Read the model definition and answer for the solid it produces. Units are mm, in the model's axes. A direction names the side the tool comes from. Coordinates: 2 decimals unless noted, no trailing zeros. Write each loop counter-clockwise with the first axis right and the second up, starting at its lowest first coordinate (ties: lowest second). Pieces come first, ordered by that corner, then holes. Notation, with made-up numbers: (-29.5, -37.5) -> (-6.5, -37.5) arc R20 cw to (-6.5, -15.5) -> close; hole circle Ø5 at (65, 37.5). An arc over 180 degrees is marked (long way). Answer as a JSON object with one key per item and string values. Group by question number.
(1) Find section A-A (z = 10.5). Give the vertices of the cut face in (x, y) (3 decimals), then the cut area to 3 significant figures.
(2) For a pull along X with two mould halves and no side action, classify faces 5 (the face through (-282.92, -76.1, 79.81)), 6 (the face through (-329.875, -83, 80)), 7 (the face through (-221.025, -83, 57)), 8 (the face through (-263.066, -87.263, 28.924)) as +X half, -X half, draft (parallel to the pull), parting line (faces both ways), or undercut.
(3) Flat-ended cylindrical pins translate along their axes: P1, Ø2, axis at y = -78, z = 43, coming from the +X side (3 decimals); P2, Ø3, axis at x = -256, y = -83, coming from the -Z side; P3, Ø15, axis at x = -290.57, z = 38.77, coming from the -Y side; P4, Ø3, axis at x = -256.5, y = -84, coming from the +Z side. Find the tip coordinate at first contact, or state that the pin passes through.
(4) Which of the six approach directions +Z, -Z, +X, -X, +Y, -Y give full straight-line access (tool end or side, diameter ignored) to faces 1 (the face through (-284, -82, 28.4)), 2 (the face through (-311, -84, 144.63)), 3 (the face through (-257, -82, 20.2)), 4 (the face through (-233.835, -87, 56))?
(5) Find section C-C (x = -275.57). Give the vertices of the cut face in (y, z).
(6) Find section D-D (z = 146.5). Give the vertices of the cut face in (x, y) (3 decimals), then the cut area to 3 significant figures.
(7) Straight lines are drawn through the part: L1, parallel to X at y = -83.75, z = 151 (3 decimals); L2, parallel to X at y = -79, z = 18 (3 decimals); L3, parallel to Z at x = -272.5, y = -84.75. For each, find the intervals that lie inside material, in ascending order.
(8) Find section B-B (x = -290.57). Give the vertices of the cut face in (y, z), then the cut area to 3 significant figures.
from build123d import *

# Parameters (mm, degrees)
SKETCH1_W           = 95.25
SKETCH1_H           = 12.8
BOSS_EXTRUDE1_DEPTH = 161.88
SKETCH1_3_R         = 3.1
CUT_EXTRUDE1_DEPTH  = 20.2
SKETCH1_4_R         = 2.395
CUT_EXTRUDE2_DEPTH  = 21.5
CUT_EXTRUDE3_REACH  = 14.8
SKETCH2_R           = 9.525
SKETCH2_R_2         = 3.265
SKETCH3_R           = 3.265
SKETCH3_R_2         = 9.525
CUT_EXTRUDE4_DEPTH  = 3.32
CUT_EXTRUDE5_START  = -17.25
SKETCH4_R           = 1.965
CUT_EXTRUDE5_DEPTH  = 17.25
SKETCH6_R           = 9.5
CUT_EXTRUDE6_DEPTH  = 13.8000001


with BuildPart() as part:
    # Sketch1 → Boss-Extrude1 (new body)
    with BuildSketch(Plane.XY):
        with Locations((-282.25, -82.5)):
            Rectangle(SKETCH1_W, SKETCH1_H)
    extrude(amount=BOSS_EXTRUDE1_DEPTH)

    # Sketch1<3> → Cut-Extrude1 (cut)
    with BuildSketch(Plane.XY):
        with Locations((-308, -82.5)):
            Circle(SKETCH1_3_R)
        with Locations((-257.2, -82.5)):
            Circle(SKETCH1_3_R)
    extrude(amount=CUT_EXTRUDE1_DEPTH, mode=Mode.SUBTRACT)

    # Sketch1<4> → Cut-Extrude2 (cut)
    with BuildSketch(Plane.XY):
        with Locations((-320.5, -82.5)):
            Circle(SKETCH1_4_R)
        with Locations((-244.2, -82.5)):
            Circle(SKETCH1_4_R)
    extrude(amount=CUT_EXTRUDE2_DEPTH, mode=Mode.SUBTRACT)

    # Sketch2 → Cut-Extrude3 (cut, up to next)
    with BuildSketch(Plane(origin=(0, -76.1, 0), x_dir=(-1, 0, 0), z_dir=(0, 1, 0)), mode=Mode.PRIVATE) as cut_extrude3_sk1:
        with Locations((275.57, 86.105)):
            Circle(SKETCH2_R)
    cut_extrude3_tool1 = extrude(cut_extrude3_sk1.sketch, amount=-CUT_EXTRUDE3_REACH, mode=Mode.PRIVATE) & part.part
    add(cut_extrude3_tool1.solids().sort_by_distance((-275.57, -76.1, 86.105))[0], mode=Mode.SUBTRACT)
    # Sketch2 → Cut-Extrude3 (cut, up to next)
    with BuildSketch(Plane(origin=(0, -76.1, 0), x_dir=(-1, 0, 0), z_dir=(0, 1, 0)), mode=Mode.PRIVATE) as cut_extrude3_sk2:
        with Locations((275.57, 124.135)):
            Circle(SKETCH2_R)
    cut_extrude3_tool2 = extrude(cut_extrude3_sk2.sketch, amount=-CUT_EXTRUDE3_REACH, mode=Mode.PRIVATE) & part.part
    add(cut_extrude3_tool2.solids().sort_by_distance((-275.57, -76.1, 124.135))[0], mode=Mode.SUBTRACT)
    # Sketch2 → Cut-Extrude3 (cut, up to next)
    with BuildSketch(Plane(origin=(0, -76.1, 0), x_dir=(-1, 0, 0), z_dir=(0, 1, 0)), mode=Mode.PRIVATE) as cut_extrude3_sk3:
        with Locations((253.55, 28.505)):
            Circle(SKETCH2_R_2)
    cut_extrude3_tool3 = extrude(cut_extrude3_sk3.sketch, amount=-CUT_EXTRUDE3_REACH, mode=Mode.PRIVATE) & part.part
    add(cut_extrude3_tool3.solids().sort_by_distance((-253.55, -76.1, 28.505))[0], mode=Mode.SUBTRACT)
    # Sketch2 → Cut-Extrude3 (cut, up to next)
    with BuildSketch(Plane(origin=(0, -76.1, 0), x_dir=(-1, 0, 0), z_dir=(0, 1, 0)), mode=Mode.PRIVATE) as cut_extrude3_sk4:
        with Locations((240.925, 140.49)):
            Circle(SKETCH2_R_2)
    cut_extrude3_tool4 = extrude(cut_extrude3_sk4.sketch, amount=-CUT_EXTRUDE3_REACH, mode=Mode.PRIVATE) & part.part
    add(cut_extrude3_tool4.solids().sort_by_distance((-240.925, -76.1, 140.49))[0], mode=Mode.SUBTRACT)
    # Sketch2 → Cut-Extrude3 (cut, up to next)
    with BuildSketch(Plane(origin=(0, -76.1, 0), x_dir=(-1, 0, 0), z_dir=(0, 1, 0)), mode=Mode.PRIVATE) as cut_extrude3_sk5:
        with BuildLine():
            Line((269.505, 25.4), (269.505, 0))
            Line((269.505, 0), (298.155, 0))
            Line((298.155, 0), (298.155, 25.4))
            ThreePointArc((298.155, 25.4), (297.276320344, 27.521320344), (295.155, 28.4))
            Line((295.155, 28.4), (272.505, 28.4))
            ThreePointArc((272.505, 28.4), (270.383679656, 27.521320344), (269.505, 25.4))
        make_face()
    cut_extrude3_tool5 = extrude(cut_extrude3_sk5.sketch, amount=-CUT_EXTRUDE3_REACH, mode=Mode.PRIVATE) & part.part
    add(cut_extrude3_tool5.solids().sort_by_distance((-283.83, -76.1, 14.135461))[0], mode=Mode.SUBTRACT)

    # Sketch3 → Cut-Extrude4 (cut)
    with BuildSketch(Plane.XZ.offset(88.9)):
        with Locations((-240.925, 140.49)):
            Circle(SKETCH3_R)
        with Locations((-253.55, 28.505)):
            Circle(SKETCH3_R_2)
    extrude(amount=-CUT_EXTRUDE4_DEPTH, mode=Mode.SUBTRACT)

    # Sketch4 → Cut-Extrude5 (cut)
    with BuildSketch(Plane.XY.offset(161.88).offset(CUT_EXTRUDE5_START)):
        with Locations((-256.825, -83.83)):
            Circle(SKETCH4_R)
        with Locations((-310.715, -83.83)):
            Circle(SKETCH4_R)
    extrude(amount=CUT_EXTRUDE5_DEPTH, mode=Mode.SUBTRACT)

    # Sketch5 → Revolve1 (revolve)
    with BuildSketch(Plane(origin=(0, -82.5, 0), x_dir=(-1, 0, 0), z_dir=(0, 1, 0))):
        with BuildLine():
            Line((234.625, 57.29), (221.025, 57.29))
            Line((221.025, 57.29), (221.025, 54.59))
            ThreePointArc((221.025, 54.59), (224.841543887, 53.18542762), (228.845807042, 52.475))
            Line((228.845807042, 52.475), (232.275807042, 52.475))
            Line((232.275807042, 52.475), (232.295, 52.925))
            Line((232.295, 52.925), (233.835, 52.925))
            Line((233.835, 52.925), (233.835, 52.09))
            Line((233.835, 52.09), (234.625, 52.09))
            Line((234.625, 52.09), (234.625, 57.29))
        make_face()
    revolve(axis=Axis((-234.625, -82.5, 57.29), (-1, 0, 0)))

    # Sketch6 → Cut-Extrude6 (cut, through all)
    with BuildSketch(Plane(origin=(0, -76.1, 0), x_dir=(-1, 0, 0), z_dir=(0, 1, 0))):
        with Locations((290.57, 38.77)):
            Circle(SKETCH6_R)
    extrude(amount=-CUT_EXTRUDE6_DEPTH, mode=Mode.SUBTRACT)


solid = part.part
Results below:
{
 "1": {"outline": "(-329.875, -88.9) -> (-298.155, -88.9) -> (-298.155, -76.1) -> (-329.875, -76.1) -> close; (-269.505, -88.9) -> (-234.625, -88.9) -> (-234.625, -76.1) -> (-269.505, -76.1) -> close; hole circle Ø4.79 at (-320.5, -82.5); hole circle Ø6.2 at (-308, -82.5); hole circle Ø6.2 at (-257.2, -82.5); hole circle Ø4.79 at (-244.2, -82.5)", "area": "756 mm2"},
 "2": {"face 5": "draft", "face 6": "-X half", "face 7": "+X half", "face 8": "undercut"},
 "3": {"P1": "stops at x = -234.625", "P2": "stops at z = 20.2", "P3": "passes through", "P4": "stops at z = 144.63"},
 "4": {"face 1": "-Z, +Y, -Y", "face 2": "+Z", "face 3": "-Z", "face 4": "none"},
 "5": {"outline": "(-88.9, 28.4) -> (-76.1, 28.4) -> (-76.1, 76.58) -> (-88.9, 76.58) -> close; (-88.9, 95.63) -> (-76.1, 95.63) -> (-76.1, 114.61) -> (-88.9, 114.61) -> close; (-88.9, 133.66) -> (-76.1, 133.66) -> (-76.1, 161.88) -> (-88.9, 161.88) -> close"},
 "6": {"outline": "(-329.875, -88.9) -> (-234.625, -88.9) -> (-234.625, -76.1) -> (-329.875, -76.1) -> close; hole circle Ø3.93 at (-310.715, -83.83); hole circle Ø3.93 at (-256.825, -83.83)", "area": "1,190 mm2"},
 "7": {"L1": "x = -329.875 to -312.678, -308.752 to -258.788, -254.862 to -234.625", "L2": "x = -329.875 to -298.155, -269.505 to -234.625", "L3": "z = 28.4 to 77.09, 95.12 to 115.12, 133.15 to 161.88"},
 "8": {"outline": "(-88.9, 28.4) -> (-76.1, 28.4) -> (-76.1, 29.27) -> (-88.9, 29.27) -> close; (-88.9, 48.27) -> (-76.1, 48.27) -> (-76.1, 161.88) -> (-88.9, 161.88) -> close", "area": "1,470 mm2"}
}
